CAD build for the part. Positions are in the model's coordinates, mm. Face numbers are marked on the shaded views. A direction names the side the tool comes from. Coordinates: 2 decimals unless noted, no trailing zeros. Order: outer loops, then holes, each group sorted by start corner. A loop starts at its lowest first (then second) coordinate and runs counter-clockwise, first axis right, second up. Notation, with made-up numbers: M -6,49.25 L -2,49.25 A20 ccw -2,78.25 Z; hole C -17.75,42 d7. An arc over 180 degrees is marked long. Write item = value, one per line. Start each with the question number.
```python
from build123d import *

# Parameters (mm, degrees)
SKETCH_1_W                       = 12.5
SKETCH_1_H                       = 25.5
SM_BASE_FLANGE_1_DEPTH           = 1.5
SM_EDGE_FLANGE_1_STRIP_W         = 7.4732
SM_EDGE_FLANGE_1_STRIP_H         = 1.5
SM_EDGE_FLANGE_1_STRIP_CUT_DEPTH = 12.5
SM_EDGE_FLANGE_1_DEPTH           = 12.5
SKETCH_6_R                       = 2.25
CUT_EXTRUDE_1_DEPTH              = 10
SKETCH_7_R                       = 2.25
CUT_EXTRUDE_2_DEPTH              = 10


# Sheet-metal steps are written as plain solids
with BuildPart() as part:
    # Sketch 1 → 基材-凸緣1 (new body)
    with BuildSketch(Plane(origin=(0, 0, 0), x_dir=(1, 0, 0), z_dir=(0, 1, 0))):
        Rectangle(SKETCH_1_W, SKETCH_1_H)
    extrude(amount=SM_BASE_FLANGE_1_DEPTH)

    # 邊線-凸緣1 strip (across the edge) → 邊線-凸緣1 strip cut (cut)
    with BuildSketch(Plane(origin=(6.25, 1.5, -12.75), x_dir=(0, 0, 1), z_dir=(-1, 0, 0))):
        with Locations((-1.5, -0.75)):
            Rectangle(SM_EDGE_FLANGE_1_STRIP_W, SM_EDGE_FLANGE_1_STRIP_H)
    extrude(amount=SM_EDGE_FLANGE_1_STRIP_CUT_DEPTH, mode=Mode.SUBTRACT)

    # 邊線-凸緣1 section (across the edge) → 邊線-凸緣1 (add)
    with BuildSketch(Plane(origin=(6.25, 1.5, -12.75), x_dir=(0, 0, 1), z_dir=(-1, 0, 0))):
        with BuildLine():
            Line((0, 0.7366), (0, 25.5))
            Line((0, 25.5), (1.5, 25.5))
            Line((1.5, 25.5), (1.5, 0.7366))
            ThreePointArc((1.5, 0.7366), (1.715745145, 0.215745145), (2.2366, 0))
            Line((2.2366, 0), (2.2366, -1.5))
            ThreePointArc((2.2366, -1.5), (0.655084973, -0.844915027), (0, 0.7366))
        make_face()
    extrude(amount=SM_EDGE_FLANGE_1_DEPTH)

    # 草圖6 → 伸長1 (cut)
    with BuildSketch(Plane(origin=(0, 1.5, 0), x_dir=(1, 0, 0), z_dir=(0, 1, 0))):
        with Locations(Location((0, -3.75, 0), (0, 0, 270))):
            Circle(SKETCH_6_R)
    extrude(amount=-CUT_EXTRUDE_1_DEPTH, mode=Mode.SUBTRACT)

    # 草圖7 → 伸長2 (cut)
    with BuildSketch(Plane.XY.offset(-11.25)):
        with Locations((0, 18)):
            Circle(SKETCH_7_R)
    extrude(amount=-CUT_EXTRUDE_2_DEPTH, mode=Mode.SUBTRACT)


solid = part.part
```
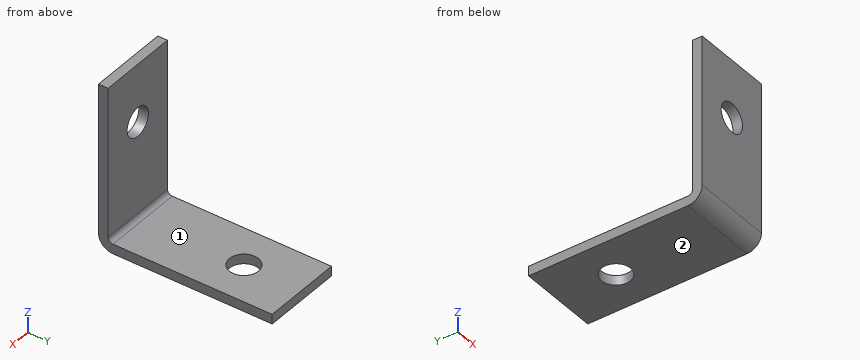
1. Slice it at B-B (y = 18). Write the cut outline in (x, z), plus the area to 3 significant figures.
2. 3-axis set-ups, long thin cutter, end or side, ignore diameter. For the marked faces 1 and 2: which of +Z, -Z, +X, -X, +Y, -Y reach the whole face in a straight line?
3. Flat gauge pins, fed straight in: pin 1 (1 mm diameter, centred on x = 3, z = -8, fed in from -Y); pin 2 (2 mm diameter, centred on x = -4.5, y = 10, fed in from +Z); pin 3 (2.5 mm diameter, centred on x = 0, y = 18, fed in from +Z). Where does each tip first touch, or does it go through?
4. Slice it at D-D (x = -3.25). Write the cut outline in (y, z), plus the area to 3 significant figures.
5. Slice it at C-C (z = 3.75). Write the cut outline in (x, y).
6. Probe L1, parallel to X at y = 0.5, z = 3.75; L2, parallel to Z at x = 0.5, y = 21.5; L3, parallel to Y at x = 3, z = 7. List the from-to ranges inside material, lowest first.
7. Slice it at A-A (x = 0). Write the cut outline in (y, z), plus the area to 3 significant figures.
Calculated:
q1.outline = M -6.25,-12.75 L -2.25,-12.75 L -2.25,-11.25 L -6.25,-11.25 Z; M 2.25,-12.75 L 6.25,-12.75 L 6.25,-11.25 L 2.25,-11.25 Z
q1.area = 12.0 mm²
q2.face_1 = +Z, +X, -X, +Y
q2.face_2 = -Z, +X, -X, +Y, -Y
q3.pin_1 = 0
q3.pin_2 = -11.25
q3.pin_3 = through
q4.outline = M 0,-10.51 A2.24 ccw 2.24,-12.75 L 27,-12.75 L 27,-11.25 L 2.24,-11.25 A0.74 cw 1.5,-10.51 L 1.5,12.75 L 0,12.75 Z
q4.area = 75.5 mm²
q5.outline = M -6.25,0 L -2.25,0 L -2.25,1.5 L -6.25,1.5 Z; M 2.25,0 L 6.25,0 L 6.25,1.5 L 2.25,1.5 Z
q6.L1 = -6.25 to -2.25, 2.25 to 6.25
q6.L2 = -12.75 to -11.25
q6.L3 = 0 to 1.5
q7.outline = M 0,-10.51 A2.24 ccw 2.24,-12.75 L 15.75,-12.75 L 15.75,-11.25 L 2.24,-11.25 A0.74 cw 1.5,-10.51 L 1.5,1.5 L 0,1.5 Z; M 0,6 L 1.5,6 L 1.5,12.75 L 0,12.75 Z; M 20.25,-12.75 L 27,-12.75 L 27,-11.25 L 20.25,-11.25 Z
q7.area = 62.0 mm²
